Design review of the part built by this model. Coordinates are the model's own, in mm. A direction names the side the tool comes from. Round coordinates to 2 decimals unless told otherwise and drop trailing zeros. Loops run counter-clockwise (first coordinate to the right, second up) from the corner with the lowest first, then second, coordinate; pieces in that order, holes last. Notation, with made-up numbers: (-3.5, 39) - (42.5, 39) arc R14 ccw to (42.5, 66) - close; hole circle Ø6 at (10.25, 52). An arc over 180 degrees is marked (long way). Return JSON: item names as keys, results as strings. Group by question number.
(1) Wall thickness on L1, parallel to X at y = 22.6, z = -3; L2, parallel to Y at x = 0, z = -5.5; L3, parallel to Z at x = -5, y = 23: over which ranges is each line inside the solid? List them lowest first. Write a range as [from, to].
(2) We need section A-A, the plane x = 0. Write out the cut boundary in (y, z), and give its area (3 significant figures).
(3) We need section D-D, the plane z = -6. Write out the cut boundary in (x, y).
(4) For faces 4 (the cylindrical face through (-2.38, -10.74, 3.2)), 5 (the flat face through (0, 25, -4)), 6 (the flat face through (-10, 19, -3)), list the 3-axis set-ups (+Z, -Z, +X, -X, +Y, -Y) from which the entire face can be reached by the end or side of a thin tool; tool diameter is ignored.
(5) Clearance check with flat-ended pins moving along their axes: pin 1 (4.5 mm diameter, centred on x = -10.5, z = -2, fed in from +Y); pin 2 (4.5 mm diameter, centred on x = -10, z = -3, fed in from -Y); pin 3 (2.5 mm diameter, centred on x = 10, z = -3, fed in from +Y); pin 4 (6.5 mm diameter, centred on x = 1.5, y = 5.5, fed in from +Z). State where each tip first meets the part, or that it passes through.
(6) We need section C-C, the plane y = 21. Write out the cut boundary in (x, z).
(7) We need section B-B, the plane z = -3. Write out the cut boundary in (x, y), and give its area (3 significant figures).
(8) The part is to be moulded in two halves that separate along Y. For faces 1 (the flat face through (5, -5, 0)), 2 (the flat face through (0, 10, -8)), 3 (the cylindrical face through (6.92, -13.31, 1.06)), say which applies: pulls with the +Y half, pulls with the -Y half, needs draft (parallel to the pull), parting line crosses it, or undercut.
from build123d import *

# Parameters (mm, degrees)
SKETCH1_R           = 15
SKETCH1_R_2         = 11
BOSS_EXTRUDE1_DEPTH = 7
BOSS_EXTRUDE2_START = 8
BOSS_EXTRUDE2_DEPTH = 8
SKETCH4_R           = 1.95
CUT_EXTRUDE1_DEPTH  = 6
SKETCH5_R           = 6
CUT_EXTRUDE2_DEPTH  = 8
CHAMFER1_SIZE       = 0.5


with BuildPart() as part:
    # Sketch1 → Boss-Extrude1 (new body)
    with BuildSketch(Plane.XY):
        Circle(SKETCH1_R)
        Circle(SKETCH1_R_2, mode=Mode.SUBTRACT)
    extrude(amount=BOSS_EXTRUDE1_DEPTH)

    # Sketch3 → Boss-Extrude2 (add)
    with BuildSketch(Plane(origin=(0, 0, 0), x_dir=(-1, 0, 0), z_dir=(0, 0, -1)).offset(BOSS_EXTRUDE2_START)):
        with BuildLine():
            Line((-15, 0), (-15, 25))
            Line((-15, 25), (15, 25))
            Line((15, 25), (15, 0))
            ThreePointArc((15, 0), (0, -15), (-15, 0))
        make_face()
    extrude(amount=-BOSS_EXTRUDE2_DEPTH)

    # Sketch4 → Cut-Extrude1 (cut)
    with BuildSketch(Plane(origin=(0, 25, 0), x_dir=(1, 0, 0), z_dir=(0, 1, 0))):
        with Locations(Location((-10, 3, 0), (0, 0, 270))):
            Circle(SKETCH4_R)
        with Locations(Location((10, 3, 0), (0, 0, 270))):
            Circle(SKETCH4_R)
    extrude(amount=-CUT_EXTRUDE1_DEPTH, mode=Mode.SUBTRACT)

    # Sketch5 → Cut-Extrude2 (cut)
    with BuildSketch(Plane.XY):
        Circle(SKETCH5_R)
    extrude(amount=-CUT_EXTRUDE2_DEPTH, mode=Mode.SUBTRACT)

    # Chamfer1
    chamfer1_edges = [part.edges().sort_by_distance(p)[0] for p in [
        (-11, 0, 7),
    ]]
    chamfer(chamfer1_edges, length=CHAMFER1_SIZE)


solid = part.part
Solutions:
{
 "1": {"L1": "[-15, -11.95], [-8.05, 8.05], [11.95, 15]", "L2": "[-15, -6], [6, 25]", "L3": "[-8, 0]"},
 "2": {"outline": "(-15, -8) - (-6, -8) - (-6, 0) - (-11, 0) - (-11, 6.5) - (-11.5, 7) - (-15, 7) - close; (6, -8) - (25, -8) - (25, 0) - (15, 0) - (15, 7) - (11.5, 7) - (11, 6.5) - (11, 0) - (6, 0) - close", "area": "280 mm^2"},
 "3": {"outline": "(-15, 0) arc R15 ccw to (15, 0) - (15, 25) - (-15, 25) - close; hole circle Ø12 at (0, 0)"},
 "4": {"face 4": "+Z", "face 5": "+Z, -Z, +X, -X, +Y", "face 6": "+Y"},
 "5": {"pin 1": "y = 25", "pin 2": "y = -12.84", "pin 3": "y = 19", "pin 4": "z = 0"},
 "6": {"outline": "(-15, -8) - (15, -8) - (15, 0) - (-15, 0) - close; hole circle Ø3.9 at (-10, -3); hole circle Ø3.9 at (10, -3)"},
 "7": {"outline": "(-15, 0) arc R15 ccw to (15, 0) - (15, 25) - (11.95, 25) - (11.95, 19) - (8.05, 19) - (8.05, 25) - (-8.05, 25) - (-8.05, 19) - (-11.95, 19) - (-11.95, 25) - (-15, 25) - close; hole circle Ø12 at (0, 0)", "area": "944 mm^2"},
 "8": {"face 1": "undercut", "face 2": "needs draft", "face 3": "parting line crosses it"}
}
